Can you work these out from the model? Positions are in its coordinate system, mm. Face numbers are marked on the shaded views. A direction names the side the tool comes from. Round coordinates to 2 decimals unless told otherwise and drop trailing zeros. Loops run counter-clockwise (first coordinate to the right, second up) from the corner with the lowest first, then second, coordinate; pieces in that order, holes last.
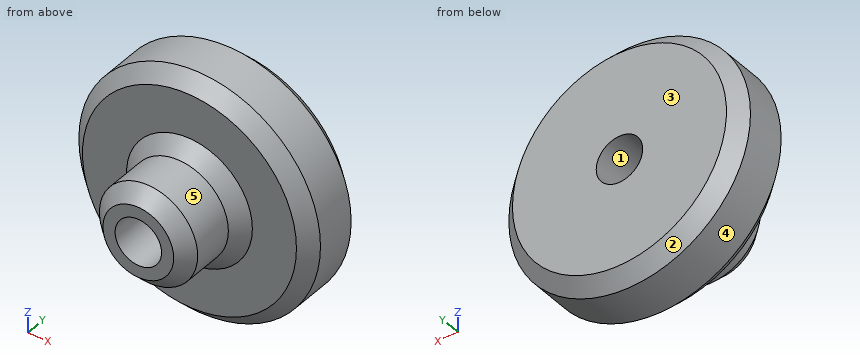
from build123d import *

# Parameters (mm, degrees)
F0_R     = 44.45
F1_DEPTH = 25.4
F2_R     = 18.07801
F3_DEPTH = 50.8
F4_R     = 8.546468
F5_DEPTH = 127
F6_SIZE  = 5.08
F7_SIZE  = 5.08


with BuildPart() as f1:
    # F0 (on Front) → F1 (new body)
    with BuildSketch(Plane.XZ):
        Circle(F0_R)
    extrude(amount=F1_DEPTH)

    # F2 (on Front) → F3 (join)
    with BuildSketch(Plane.XZ):
        Circle(F2_R)
    extrude(amount=F3_DEPTH)

    # F4 (on face) → F5 (cut)
    with BuildSketch(Plane.XZ.offset(50.8)):
        Circle(F4_R)
    extrude(amount=-F5_DEPTH, mode=Mode.SUBTRACT)

    # F6
    f6_edges = [f1.edges().sort_by_distance(p)[0] for p in [
        (-18.07801, -25.4, 0),
        (18.07801, -38.1, 0),
        (-18.07801, -50.8, 0),
    ]]
    chamfer(f6_edges, length=F6_SIZE)

    # F7
    f7_edges = [f1.edges().sort_by_distance(p)[0] for p in [
        (44.45, -12.7, 0),
        (-44.45, 0, 0),
        (-44.45, -25.4, 0),
    ]]
    chamfer(f7_edges, length=F7_SIZE)


solid = f1.part
(1) If we section it at D-D, the plane y = -23: List the corners of the cut face in (x, z) for me.
Worked answers:
outline: circle Ø83.54 at (0, 0); hole circle Ø17.09 at (0, 0)
(2) If we section it at C-C, the plane y = -17: List the corners of the cut face in (x, z) for me, then the cut area to 3 significant figures.
Worked answers:
outline: circle Ø88.9 at (0, 0); hole circle Ø17.09 at (0, 0)
area: 5,980 mm2
(3) If we section it at A-A, the plane x = 0: List the corners of the cut face in (y, z) for me.
Worked answers:
outline: (-50.8, -13) - (-45.72, -18.08) - (-30.48, -18.08) - (-25.4, -23.16) - (-25.4, -39.37) - (-20.32, -44.45) - (-5.08, -44.45) - (0, -39.37) - (0, -8.55) - (-50.8, -8.55) - close; (-50.8, 8.55) - (0, 8.55) - (0, 39.37) - (-5.08, 44.45) - (-20.32, 44.45) - (-25.4, 39.37) - (-25.4, 23.16) - (-30.48, 18.08) - (-45.72, 18.08) - (-50.8, 13) - close
(4) If we mould it in two halves opening along Z, with no side actions, what happens to the marked faces 1, 2 and 3? For each: released by +Z, released by -Z, zero draft, split by the parting line, or undercut.
Worked answers:
face 1: undercut
face 2: split by the parting line
face 3: zero draft
(5) For the marked faces 4 and 5, which set-ups out of +Z, -Z, +X, -X, +Y, -Y let a thin tool reach every point of the face, with its end or its side?
Worked answers:
face 4: +Y, -Y
face 5: -Y
(6) Will these pins go through, and if not, where does the flat tip stop? P1, Ø1.5, axis at y = -24, z = 29.5, coming from the +X side; P2, Ø6, axis at x = -5.5, y = -36.5, coming from the +Z side; P3, Ø12, axis at y = -40.5, z = 9.5, coming from the +X side.
Worked answers:
P1: stops at x = 29.46
P2: stops at z = 17.9
P3: stops at x = 17.74
(7) If I drill on line 1 (Z direction, x = 0, y = -32.5); line 2 (Z direction, x = 0, y = -17.5); line 3 (Y direction, x = -18.5, z = -28.5), over which ranges is the centre line in solid material (lowest first)?
Worked answers:
line 1: z = -18.08 to -8.55, 8.55 to 18.08
line 2: z = -44.45 to -8.55, 8.55 to 44.45
line 3: y = -25.4 to 0
(8) If we section it at B-B, the plane z = 0: List the corners of the cut face in (x, y) for me, then the cut area to 3 significant figures.
Worked answers:
outline: (-44.45, -20.32) - (-39.37, -25.4) - (-23.16, -25.4) - (-18.08, -30.48) - (-18.08, -45.72) - (-13, -50.8) - (-8.55, -50.8) - (-8.55, 0) - (-39.37, 0) - (-44.45, -5.08) - close; (8.55, -50.8) - (13, -50.8) - (18.08, -45.72) - (18.08, -30.48) - (23.16, -25.4) - (39.37, -25.4) - (44.45, -20.32) - (44.45, -5.08) - (39.37, 0) - (8.55, 0) - close
area: 2,260 mm2
